The listing builds one solid part. Answer for the finished solid, in the listing's coordinates (mm). Face numbers are marked on the shaded views. A direction names the side the tool comes from. Coordinates: 2 decimals unless noted, no trailing zeros. Write each loop counter-clockwise with the first axis right and the second up, starting at its lowest first coordinate (ties: lowest second). Pieces come first, ordered by that corner, then holes. Notation, with made-up numbers: M -28.75,-3.5 L -2.75,-3.5 A23 ccw -2.75,11.5 Z; hole C 31,25.25 d9. An arc over 180 degrees is marked long. Answer as CSV lines item,"result". Start each with the question number.
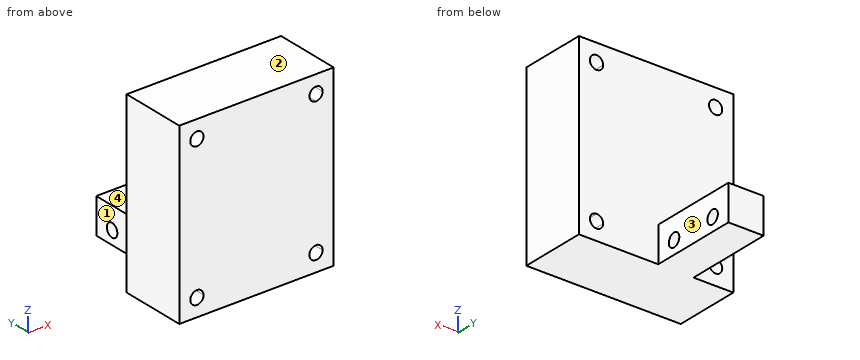
```python
from build123d import *

# Parameters (mm, degrees)
SKETCH_1_W          = 35
SKETCH_1_H          = 40
EXTRUDE_1_DEPTH     = 15
SKETCH_4_R          = 1.5
CUT_EXTRUDE_1_DEPTH = 25
SKETCH_5_W          = 8
SKETCH_5_H          = 8
EXTRUDE_2_DEPTH     = 20
SKETCH_6_R          = 1.5
CUT_EXTRUDE_2_DEPTH = 20


with BuildPart() as part:
    # Эскиз1 → Бобышка-Вытянуть1 (new body)
    with BuildSketch(Plane(origin=(0, 0, 0), x_dir=(1, 0, 0), z_dir=(0, 1, 0))):
        Rectangle(SKETCH_1_W, SKETCH_1_H)
    extrude(amount=EXTRUDE_1_DEPTH)

    # Эскиз4 → Вырез-Вытянуть1 (cut)
    with BuildSketch(Plane(origin=(0, 15, 0), x_dir=(1, 0, 0), z_dir=(0, 1, 0))):
        with BuildLine():
            ThreePointArc((-12, 16), (-14.560660172, 17.060660172), (-13.5, 14.5))
            Line((-13.5, 14.5), (-13.5, 16))
            Line((-13.5, 16), (-12, 16))
        make_face()
        with BuildLine():
            Line((-13.5, 16), (-13.5, 14.5))
            ThreePointArc((-13.5, 14.5), (-12.439339828, 14.939339828), (-12, 16))
            Line((-12, 16), (-13.5, 16))
        make_face()
        with BuildLine():
            ThreePointArc((15, -16), (14.560660172, -14.939339828), (13.5, -14.5))
            Line((13.5, -14.5), (13.5, -16))
            Line((13.5, -16), (12, -16))
            ThreePointArc((12, -16), (13.5, -17.5), (15, -16))
        make_face()
        with BuildLine():
            Line((13.5, -16), (13.5, -14.5))
            ThreePointArc((13.5, -14.5), (12.439339828, -14.939339828), (12, -16))
            Line((12, -16), (13.5, -16))
        make_face()
        with BuildLine():
            ThreePointArc((12, 16), (12.439339828, 14.939339828), (13.5, 14.5))
            Line((13.5, 14.5), (13.5, 16))
            Line((13.5, 16), (12, 16))
        make_face()
        with BuildLine():
            Line((13.5, 16), (13.5, 14.5))
            ThreePointArc((13.5, 14.5), (14.560660172, 14.939339828), (15, 16))
            ThreePointArc((15, 16), (13.5, 17.5), (12, 16))
            Line((12, 16), (13.5, 16))
        make_face()
        with Locations((-13.5, -16)):
            Circle(SKETCH_4_R)
    extrude(amount=-CUT_EXTRUDE_1_DEPTH, mode=Mode.SUBTRACT)

    # Эскиз5 → Бобышка-Вытянуть2 (add)
    with BuildSketch(Plane(origin=(0, 15, 0), x_dir=(1, 0, 0), z_dir=(0, 1, 0))):
        with Locations((-4.5, 16)):
            Rectangle(SKETCH_5_W, SKETCH_5_H)
    extrude(amount=EXTRUDE_2_DEPTH)

    # Эскиз6 → Вырез-Вытянуть2 (cut)
    with BuildSketch(Plane(origin=(-0.5, 0, 0), x_dir=(0, 0, -1), z_dir=(1, 0, 0))):
        with Locations((17, 30.5)):
            Circle(SKETCH_6_R)
        with Locations((17, 19.5)):
            Circle(SKETCH_6_R)
    extrude(amount=-CUT_EXTRUDE_2_DEPTH, mode=Mode.SUBTRACT)


solid = part.part
```
1) The part is cut by section A-A (y = 30.5). Determine the outline of the cut face in (x, z), then the cut area to 3 significant figures.
2) Find the intervals of material crossed by line 1 (Y direction, x = -2, z = -17); line 2 (X direction, y = 4, z = -16); line 3 (Y direction, x = 4.5, z = -14), in increasing order. Write a range as from..to.
3) The part is cut by section B-B (y = 4). Determine the outline of the cut face in (x, z), then the cut area to 3 significant figures.
4) Which of the six approach directions +Z, -Z, +X, -X, +Y, -Y give full straight-line access (tool end or side, diameter ignored) to the marked faces 1, 2, 3 and 4?
5) The part is cut by section C-C (z = 4). Determine the outline of the cut face in (x, y), then the cut area to 3 significant figures.
6) Each of these flat-tipped pins is pushed along its axis until it touches: P1, Ø1, axis at x = -8, z = 0, coming from the +Y side; P2, Ø6.5, axis at x = -5, y = 21.5, coming from the +Z side; P3, Ø6, axis at x = 4.5, y = 27, coming from the +Z side; P4, Ø9, axis at y = 28, z = -15.5, coming from the -X side. Where does it stop, or does it pass through?
7) The part is cut by section D-D (y = 26.5). Determine the outline of the cut face in (x, z).
Completed:
1,outline,"M -8.5,-20 L -0.5,-20 L -0.5,-18.5 L -8.5,-18.5 Z; M -8.5,-15.5 L -0.5,-15.5 L -0.5,-12 L -8.5,-12 Z"
1,area,"40.0 mm²"
2,line 1,"0..18, 21..29, 32..35"
2,line 2,"-17.5..-15, -12..12, 15..17.5"
2,line 3,"0..15"
3,outline,"M -17.5,-20 L 17.5,-20 L 17.5,20 L -17.5,20 Z; hole C -13.5,-16 d3; hole C -13.5,16 d3; hole C 13.5,-16 d3; hole C 13.5,16 d3"
3,area,"1,370 mm²"
4,face 1,"+Z, -Z, -X, +Y"
4,face 2,"+Z, +X, -X, +Y, -Y"
4,face 3,"+Z, -Z, +X, +Y"
4,face 4,"+Z, +X, -X, +Y"
5,outline,"M -17.5,0 L 17.5,0 L 17.5,15 L -17.5,15 Z"
5,area,"525 mm²"
6,P1,"y = 15"
6,P2,"z = -12"
6,P3,"through"
6,P4,"x = -8.5"
7,outline,"M -8.5,-20 L -0.5,-20 L -0.5,-12 L -8.5,-12 Z"
